```python
from build123d import *

# Parameters (mm, degrees)
F0_W     = 60
F0_H     = 50
F0_W_2   = 60.0000097896
F1_DEPTH = 25
F2_R     = 5


# Not quite as in the source:
# - ends of sketch curves that miss each other by under 0.0002 mm in the source are joined


with BuildPart() as f1:
    # F0 (on Top) → F1 (new body)
    with BuildSketch(Plane.XY):
        with Locations((-140, 0)):
            Rectangle(F0_W, F0_H)
        with BuildLine():
            Line((-110, 25), (-110, -25))
            ThreePointArc((-110, -25), (-4.8948e-06, -15), (109.9999902104, -25))
            Line((109.9999902104, -25), (109.9999902104, 25))
            ThreePointArc((109.9999902104, 25), (0, 14.9999991026), (-110, 25))
        make_face()
        with Locations((139.9999951052, 0)):
            Rectangle(F0_W_2, F0_H)
    extrude(amount=F1_DEPTH)

    # F2
    f2_edges = [f1.edges().sort_by_distance(p)[0] for p in [
        (-140, -25, 25),
        (-5e-06, -15, 25),
        (139.999995, -25, 25),
        (139.999995, 25, 25),
        (-5e-06, 14.999999, 25),
        (-140, 25, 25),
        (-140, -25, 0),
        (-5e-06, -15, 0),
        (139.999995, -25, 0),
        (-140, 25, 0),
        (-5e-06, 14.999999, 0),
        (139.999995, 25, 0),
    ]]
    fillet(f2_edges, radius=F2_R)


solid = f1.part
```
CAD build for the part. Positions are in the model's coordinates, mm. Round coordinates to 2 decimals unless told otherwise and drop trailing zeros. Write each loop counter-clockwise with the first axis right and the second up, starting at its lowest first coordinate (ties: lowest second). Pieces come first, ordered by that corner, then holes. Notation, with made-up numbers: (62.25, -33) - (116.25, -33) arc R10 cw to (116.25, -25) - close; hole circle Ø8 at (63.5, 49.5). An arc over 180 degrees is marked (long way). Return JSON: item names as keys, results as strings. Group by question number.
Item 1: Band-saw the part on B-B on x = -135. List the corners of the cut face in (y, z).
Item 2: Probe probe 1 along Y at (x, z) = (2, 15); probe 2 along Y at (x, z) = (11.5, 20); probe 3 along Z at (x, y) = (-40.5, -14). List the from-to ranges inside material, lowest first.
Item 3: Flat gauge pins, fed straight in: pin 1 Ø1.5 at (x, y) = (90, 17) entering from -Z; pin 2 Ø10 at (x, z) = (-89, 13) entering from -Y; pin 3 Ø5 at (x, z) = (65, 14.5) entering from -Y. Where does each tip first touch, or does it go through?
Item 4: Mould opens along X. For faces 1 (the face through (-170, 0, 12)), 2 (the face through (1.5, 15, 12.4)), 3 (the face through (-140, -25, 12)), 4 (the face through (-1.5, -15, 12.4)) say: +X half, -X half, draft (parallel to the pull), parting line (faces both ways), or undercut.
Item 5: Band-saw the part on A-A on z = 16.5. List the corners of the cut face in (x, y).
Resolved:
{
 "1": {"outline": "(-25, 5) arc R5 ccw to (-20, 0) - (20, 0) arc R5 ccw to (25, 5) - (25, 20) arc R5 ccw to (20, 25) - (-20, 25) arc R5 ccw to (-25, 20) - close"},
 "2": {"probe 1": "y = -15 to 15", "probe 2": "y = -15.11 to 15.11", "probe 3": "z = 0.77 to 24.23"},
 "3": {"pin 1": "stops at z = 0", "pin 2": "stops at y = -22.29", "pin 3": "stops at y = -18.75"},
 "4": {"face 1": "-X half", "face 2": "undercut", "face 3": "draft", "face 4": "undercut"},
 "5": {"outline": "(-170, -25) - (-110, -25) arc R610 cw to (110, -25) - (170, -25) - (170, 25) - (110, 25) arc R610 cw to (-110, 25) - (-170, 25) - close"}
}
